from build123d import *

# Parameters (mm, degrees)
F0_W     = 101.4476
F0_H     = 101.5520170331
F1_DEPTH = 152.4
F5_D     = 11.50874
F6_D     = 13.1064
F6_DEPTH = 101.6
F6_TIP   = 3.9375598086
F7_D     = 6.5278
F7_DEPTH = 101.6
F7_TIP   = 1.9611489744


with BuildPart() as f1:
    # F0 (on Front) → F1 (new body)
    with BuildSketch(Plane.XZ):
        with Locations((50.7238, -50.7760085166)):
            Rectangle(F0_W, F0_H)
    extrude(amount=F1_DEPTH)

    # F5 (through all)
    with Locations(Plane(origin=(0, 0, 0), x_dir=(-1, 0, 0), z_dir=(0, 1, 0))):
        with Locations((-76.6532495618, -47.2862608731), (-24.7153807431, -49.5884530246)):
            Hole(F5_D / 2)

    # F6
    with Locations(Plane(origin=(0, 0, 0), x_dir=(-1, 0, 0), z_dir=(0, 1, 0))):
        with Locations((-51.1274710298, -21.4095711708)):
            Hole(F6_D / 2, depth=F6_DEPTH)
            with Locations((0, 0, -(F6_DEPTH + F6_TIP / 2))):  # 118° drill point
                Cone(0, F6_D / 2, F6_TIP, mode=Mode.SUBTRACT)

    # F7
    with Locations(Plane(origin=(0, 0, 0), x_dir=(-1, 0, 0), z_dir=(0, 1, 0))):
        with Locations((-50.2411611378, -75.4651352763)):
            Hole(F7_D / 2, depth=F7_DEPTH)
            with Locations((0, 0, -(F7_DEPTH + F7_TIP / 2))):  # 118° drill point
                Cone(0, F7_D / 2, F7_TIP, mode=Mode.SUBTRACT)


solid = f1.part
Read the model definition and answer for the solid it produces. Units are mm, in the model's axes. A direction names the side the tool comes from. Round coordinates to 2 decimals unless told otherwise and drop trailing zeros. Order: outer loops, then holes, each group sorted by start corner. A loop starts at its lowest first (then second) coordinate and runs counter-clockwise, first axis right, second up.
1) The part is cut by section D-D on y = -48. Write down the section's boundary in (x, z).
2) The part is cut by section C-C on x = 74.5. Write down the section's boundary in (y, z), plus the area to 4 significant figures.
3) The part is cut by section A-A on x = 27.5. Write down the section's boundary in (y, z).
4) The part is cut by section B-B on y = -136.5. Write down the section's boundary in (x, z).
5) The mould has two halves that part along Z. Classify faces 1 (the face through (50, -75, 0)), 2 (the face through (50, 0, -50)), 3 (the face through (52.264, -104.854, -21.36)): released by +Z, released by -Z, zero draft, split by the parting line, or undercut.
6) For faces 4 (the face through (50, -152.4, -50)), 5 (the face through (49.707, -51.511, -27.807)), determine the directions among +Z, -Z, +X, -X, +Y, -Y from which every point of the face is accessible in a straight line to the end or side of a thin tool.
7) Straight lines are drawn through the part: L1, parallel to Z at x = 76, y = -70.5; L2, parallel to Z at x = 81.5, y = -42; L3, parallel to X at y = -31, z = -48. For each, find the intervals that lie inside material, in ascending order.
Resolved:
1. outline: (0, -101.55) - (101.45, -101.55) - (101.45, 0) - (0, 0) - close; hole circle Ø11.51 at (24.72, -49.59); hole circle Ø13.11 at (51.13, -21.41); hole circle Ø6.53 at (50.24, -75.47); hole circle Ø11.51 at (76.65, -47.29)
2. outline: (-152.4, -101.55) - (0, -101.55) - (0, -52.62) - (-152.4, -52.62) - close; (-152.4, -41.95) - (0, -41.95) - (0, 0) - (-152.4, 0) - close
2. area: 13,850 mm2
3. outline: (-152.4, -101.55) - (0, -101.55) - (0, -54.62) - (-152.4, -54.62) - close; (-152.4, -44.55) - (0, -44.55) - (0, 0) - (-152.4, 0) - close
4. outline: (0, -101.55) - (101.45, -101.55) - (101.45, 0) - (0, 0) - close; hole circle Ø11.51 at (24.72, -49.59); hole circle Ø11.51 at (76.65, -47.29)
5. face 1: released by +Z
5. face 2: zero draft
5. face 3: undercut
6. face 4: +Z, -Z, +X, -X, -Y
6. face 5: +Y
7. L1: z = -101.55 to -53, -41.57 to 0
7. L2: z = -101.55 to -50.39, -44.18 to 0
7. L3: x = 0 to 19.18, 30.25 to 70.94, 82.36 to 101.45
